For this review, take the finished solid that the model builds, in its own axes (mm). Give positions to 0.01 mm unless a question says otherwise; leave off trailing zeros. Loops run counter-clockwise (first coordinate to the right, second up) from the corner with the lowest first, then second, coordinate; pieces in that order, holes last. Notation, with made-up numbers: (49, 48) -> (55, 48) arc R20 cw to (55, 77) -> close; hole circle Ø11 at (78.5, 19). An arc over 180 degrees is marked (long way). Write each question's results on one line, items separated by ' | '. Start each with the question number.
```python
from build123d import *

# Parameters (mm, degrees)
F1_DEPTH = 60
F2_DEPTH = 50
F3_R     = 39
F4_DEPTH = 10
F3_R_2   = 49
F5_DEPTH = 3
F6_D     = 4
F6_DEPTH = 20
F6_TIP   = 1.2017212381


with BuildPart() as f1:
    # F0 (on Top) → F1 (new body, symmetric)
    with BuildSketch(Plane.XY):
        with BuildLine():
            ThreePointArc((-20.6806279512, -212.5965936405), (-39.6511040787, -210.0990830779), (-51.299249736, -194.9189241108))
            Line((-51.299249736, -194.9189241108), (-96.5925826289, -25.8819045103))
            ThreePointArc((-96.5925826289, -25.8819045103), (-96.7999862455, -25.034315887), (-96.9702211634, -24.1784871615))
            Line((-96.9702211634, -24.1784871615), (-59.4134556551, -237.1734885924))
            ThreePointArc((-59.4134556551, -237.1734885924), (-58.8379861015, -234.2804077793), (-56.4591683744, -232.5361864574))
            Line((-56.4591683744, -232.5361864574), (54.3519994715, -202.8444235207))
            ThreePointArc((54.3519994715, -202.8444235207), (60.4240630584, -198.1851652578), (61.4230672834, -190.5969748068))
            Line((61.4230672834, -190.5969748068), (52.3644007048, -156.7895708867))
            ThreePointArc((52.3644007048, -156.7895708867), (50.8658943672, -168.1718565632), (41.757798987, -175.1607439575))
            Line((41.757798987, -175.1607439575), (-25.8570088532, -193.2780771147))
            ThreePointArc((-25.8570088532, -193.2780771147), (-31.9807332102, -189.7425432088), (-28.4451993043, -183.6188188518))
            Line((-28.4451993043, -183.6188188518), (39.169608536, -165.5014856947))
            ThreePointArc((39.169608536, -165.5014856947), (49.7762102538, -147.1303126238), (31.4050371829, -136.523710906))
            Line((31.4050371829, -136.523710906), (-36.2097706573, -154.6410440632))
            ThreePointArc((-36.2097706573, -154.6410440632), (-42.3334950143, -151.1055101572), (-38.7979611084, -144.9817858003))
            Line((-38.7979611084, -144.9817858003), (28.8168467319, -126.8644526431))
            ThreePointArc((28.8168467319, -126.8644526431), (37.9249421121, -119.8755652488), (39.4234484497, -108.4932795722))
            Line((39.4234484497, -108.4932795722), (9.6592582629, 2.588190451))
            ThreePointArc((9.6592582629, 2.588190451), (5, 8.6602540378), (-2.588190451, 9.6592582629))
            Line((-2.588190451, 9.6592582629), (-79.8622565541, -11.0462653453))
            ThreePointArc((-79.8622565541, -11.0462653453), (-85.934320141, -15.7055236082), (-86.933324366, -23.2937140592))
            Line((-86.933324366, -23.2937140592), (-61.0514198558, -119.8862966881))
            ThreePointArc((-61.0514198558, -119.8862966881), (-56.3921615929, -125.958360275), (-48.8039711418, -126.9573645))
            Line((-48.8039711418, -126.9573645), (23.6404658298, -107.5459361173))
            ThreePointArc((23.6404658298, -107.5459361173), (29.7641901868, -111.0814700232), (26.2286562809, -117.2051943802))
            Line((26.2286562809, -117.2051943802), (-41.3861515594, -135.3225275374))
            ThreePointArc((-41.3861515594, -135.3225275374), (-51.9927532772, -153.6937006083), (-33.6215802063, -164.300302326))
            Line((-33.6215802063, -164.300302326), (33.9932276339, -146.1829691689))
            ThreePointArc((33.9932276339, -146.1829691689), (40.1169519909, -149.7185030748), (36.581418085, -155.8422274318))
            Line((36.581418085, -155.8422274318), (-31.0333897553, -173.9595605889))
            ThreePointArc((-31.0333897553, -173.9595605889), (-41.6399914731, -192.3307336598), (-23.2688184022, -202.9373353776))
            Line((-23.2688184022, -202.9373353776), (44.345989438, -184.8200022204))
            ThreePointArc((44.345989438, -184.8200022204), (50.469713795, -188.3555361264), (46.9341798891, -194.4792604833))
            Line((46.9341798891, -194.4792604833), (-20.6806279512, -212.5965936405))
        make_face()
        with BuildLine():
            Line((-96.5925826289, -25.8819045103), (-51.299249736, -194.9189241108))
            ThreePointArc((-51.299249736, -194.9189241108), (-39.6511040787, -210.0990830779), (-20.6806279512, -212.5965936405))
            Line((-20.6806279512, -212.5965936405), (46.9341798891, -194.4792604833))
            ThreePointArc((46.9341798891, -194.4792604833), (50.469713795, -188.3555361264), (44.345989438, -184.8200022204))
            Line((44.345989438, -184.8200022204), (-23.2688184022, -202.9373353776))
            ThreePointArc((-23.2688184022, -202.9373353776), (-41.6399914731, -192.3307336598), (-31.0333897553, -173.9595605889))
            Line((-31.0333897553, -173.9595605889), (36.581418085, -155.8422274318))
            ThreePointArc((36.581418085, -155.8422274318), (40.1169519909, -149.7185030748), (33.9932276339, -146.1829691689))
            Line((33.9932276339, -146.1829691689), (-33.6215802063, -164.300302326))
            ThreePointArc((-33.6215802063, -164.300302326), (-51.9927532772, -153.6937006083), (-41.3861515594, -135.3225275374))
            Line((-41.3861515594, -135.3225275374), (26.2286562809, -117.2051943802))
            ThreePointArc((26.2286562809, -117.2051943802), (29.7641901868, -111.0814700232), (23.6404658298, -107.5459361173))
            Line((23.6404658298, -107.5459361173), (-48.8039711418, -126.9573645))
            ThreePointArc((-48.8039711418, -126.9573645), (-56.3921615929, -125.958360275), (-61.0514198558, -119.8862966881))
            Line((-61.0514198558, -119.8862966881), (-86.933324366, -23.2937140592))
            ThreePointArc((-86.933324366, -23.2937140592), (-85.934320141, -15.7055236082), (-79.8622565541, -11.0462653453))
            Line((-79.8622565541, -11.0462653453), (-2.588190451, 9.6592582629))
            ThreePointArc((-2.588190451, 9.6592582629), (5, 8.6602540378), (9.6592582629, 2.588190451))
            Line((9.6592582629, 2.588190451), (39.4234484497, -108.4932795722))
            ThreePointArc((39.4234484497, -108.4932795722), (37.9249421121, -119.8755652488), (28.8168467319, -126.8644526431))
            Line((28.8168467319, -126.8644526431), (-38.7979611084, -144.9817858003))
            ThreePointArc((-38.7979611084, -144.9817858003), (-42.3334950143, -151.1055101572), (-36.2097706573, -154.6410440632))
            Line((-36.2097706573, -154.6410440632), (31.4050371829, -136.523710906))
            ThreePointArc((31.4050371829, -136.523710906), (49.7762102538, -147.1303126238), (39.169608536, -165.5014856947))
            Line((39.169608536, -165.5014856947), (-28.4451993043, -183.6188188518))
            ThreePointArc((-28.4451993043, -183.6188188518), (-31.9807332102, -189.7425432088), (-25.8570088532, -193.2780771147))
            Line((-25.8570088532, -193.2780771147), (41.757798987, -175.1607439575))
            ThreePointArc((41.757798987, -175.1607439575), (50.8658943672, -168.1718565632), (52.3644007048, -156.7895708867))
            Line((52.3644007048, -156.7895708867), (61.4230672834, -190.5969748068))
            ThreePointArc((61.4230672834, -190.5969748068), (60.4240630584, -198.1851652578), (54.3519994715, -202.8444235207))
            Line((54.3519994715, -202.8444235207), (-56.4591683744, -232.5361864574))
            ThreePointArc((-56.4591683744, -232.5361864574), (-58.8379861015, -234.2804077793), (-59.4134556551, -237.1734885924))
            ThreePointArc((-59.4134556551, -237.1734885924), (-58.0216629892, -239.5841442033), (-55.4059483937, -240.5361864574))
            Line((-55.4059483937, -240.5361864574), (30.7766323053, -240.5361864574))
            ThreePointArc((30.7766323053, -240.5361864574), (63.8813029697, -224.210769539), (71.0823255463, -188.0087843558))
            Line((71.0823255463, -188.0087843558), (19.3185165258, 5.1763809021))
            ThreePointArc((19.3185165258, 5.1763809021), (10, 17.3205080757), (-5.1763809021, 19.3185165258))
            Line((-5.1763809021, 19.3185165258), (-82.4504470052, -1.3870070824))
            ThreePointArc((-82.4504470052, -1.3870070824), (-94.1418950194, -9.9595314413), (-96.9702211634, -24.1784871615))
            ThreePointArc((-96.9702211634, -24.1784871615), (-96.7999862455, -25.034315887), (-96.5925826289, -25.8819045103))
        make_face()
    extrude(amount=F1_DEPTH, both=True)

    # F0 (on Top) → F2 (cut, symmetric)
    with BuildSketch(Plane.XY):
        with BuildLine():
            ThreePointArc((-20.6806279512, -212.5965936405), (-39.6511040787, -210.0990830779), (-51.299249736, -194.9189241108))
            Line((-51.299249736, -194.9189241108), (-96.5925826289, -25.8819045103))
            ThreePointArc((-96.5925826289, -25.8819045103), (-96.7999862455, -25.034315887), (-96.9702211634, -24.1784871615))
            Line((-96.9702211634, -24.1784871615), (-59.4134556551, -237.1734885924))
            ThreePointArc((-59.4134556551, -237.1734885924), (-58.8379861015, -234.2804077793), (-56.4591683744, -232.5361864574))
            Line((-56.4591683744, -232.5361864574), (54.3519994715, -202.8444235207))
            ThreePointArc((54.3519994715, -202.8444235207), (60.4240630584, -198.1851652578), (61.4230672834, -190.5969748068))
            Line((61.4230672834, -190.5969748068), (52.3644007048, -156.7895708867))
            ThreePointArc((52.3644007048, -156.7895708867), (50.8658943672, -168.1718565632), (41.757798987, -175.1607439575))
            Line((41.757798987, -175.1607439575), (-25.8570088532, -193.2780771147))
            ThreePointArc((-25.8570088532, -193.2780771147), (-31.9807332102, -189.7425432088), (-28.4451993043, -183.6188188518))
            Line((-28.4451993043, -183.6188188518), (39.169608536, -165.5014856947))
            ThreePointArc((39.169608536, -165.5014856947), (49.7762102538, -147.1303126238), (31.4050371829, -136.523710906))
            Line((31.4050371829, -136.523710906), (-36.2097706573, -154.6410440632))
            ThreePointArc((-36.2097706573, -154.6410440632), (-42.3334950143, -151.1055101572), (-38.7979611084, -144.9817858003))
            Line((-38.7979611084, -144.9817858003), (28.8168467319, -126.8644526431))
            ThreePointArc((28.8168467319, -126.8644526431), (37.9249421121, -119.8755652488), (39.4234484497, -108.4932795722))
            Line((39.4234484497, -108.4932795722), (9.6592582629, 2.588190451))
            ThreePointArc((9.6592582629, 2.588190451), (5, 8.6602540378), (-2.588190451, 9.6592582629))
            Line((-2.588190451, 9.6592582629), (-79.8622565541, -11.0462653453))
            ThreePointArc((-79.8622565541, -11.0462653453), (-85.934320141, -15.7055236082), (-86.933324366, -23.2937140592))
            Line((-86.933324366, -23.2937140592), (-61.0514198558, -119.8862966881))
            ThreePointArc((-61.0514198558, -119.8862966881), (-56.3921615929, -125.958360275), (-48.8039711418, -126.9573645))
            Line((-48.8039711418, -126.9573645), (23.6404658298, -107.5459361173))
            ThreePointArc((23.6404658298, -107.5459361173), (29.7641901868, -111.0814700232), (26.2286562809, -117.2051943802))
            Line((26.2286562809, -117.2051943802), (-41.3861515594, -135.3225275374))
            ThreePointArc((-41.3861515594, -135.3225275374), (-51.9927532772, -153.6937006083), (-33.6215802063, -164.300302326))
            Line((-33.6215802063, -164.300302326), (33.9932276339, -146.1829691689))
            ThreePointArc((33.9932276339, -146.1829691689), (40.1169519909, -149.7185030748), (36.581418085, -155.8422274318))
            Line((36.581418085, -155.8422274318), (-31.0333897553, -173.9595605889))
            ThreePointArc((-31.0333897553, -173.9595605889), (-41.6399914731, -192.3307336598), (-23.2688184022, -202.9373353776))
            Line((-23.2688184022, -202.9373353776), (44.345989438, -184.8200022204))
            ThreePointArc((44.345989438, -184.8200022204), (50.469713795, -188.3555361264), (46.9341798891, -194.4792604833))
            Line((46.9341798891, -194.4792604833), (-20.6806279512, -212.5965936405))
        make_face()
    extrude(amount=F2_DEPTH, both=True, mode=Mode.SUBTRACT)

    # F3 (on face) → F4 (cut)
    with BuildSketch(Plane(origin=(19.3185165258, 5.1763809021, 0), x_dir=(-0.2588190451, 0.9659258263, 0), z_dir=(0.9659258263, 0.2588190451, 0))):
        with Locations((-55, 0)):
            Circle(F3_R)
    extrude(amount=-F4_DEPTH, mode=Mode.SUBTRACT)

    # F3 (on face) → F5 (cut)
    with BuildSketch(Plane(origin=(19.3185165258, 5.1763809021, 0), x_dir=(-0.2588190451, 0.9659258263, 0), z_dir=(0.9659258263, 0.2588190451, 0))):
        with Locations((-55, 0)):
            Circle(F3_R_2)
        with Locations((-55, 0)):
            Circle(F3_R, mode=Mode.SUBTRACT)
    extrude(amount=-F5_DEPTH, mode=Mode.SUBTRACT)

    # F6
    with Locations(Plane(origin=(19.3185165258, 5.1763809021, 0), x_dir=(-0.2588190451, 0.9659258263, 0), z_dir=(0.9659258263, 0.2588190451, 0))):
        with Locations((-10, 0), (-32.5, -38.9711431703), (-77.5, -38.9711431703), (-100, 0), (-77.5, 38.9711431703), (-32.5, 38.9711431703)):
            Hole(F6_D / 2, depth=F6_DEPTH)
            with Locations((0, 0, -(F6_DEPTH + F6_TIP / 2))):  # 118° drill point
                Cone(0, F6_D / 2, F6_TIP, mode=Mode.SUBTRACT)


solid = f1.part
```
1. We need section C-C (y = -150). Write out the cut boundary in (x, z), plus the area to 3 significant figures.
2. We need section A-A (x = -16). Write out the cut boundary in (y, z).
3. Draft analysis for pull direction X (two halves, no side actions). For faces 1 (the cylindrical face through (28.64, -54.52, 38.67)), 2 (the flat face through (-14, -108, -60)), 3 (the flat face through (51.314, -114.234, 0.84)), state which applies: released by +X, released by -X, zero draft, split by the parting line, or undercut.
4. Wall thickness on L1, parallel to Z at x = -46.5, y = -157.5; L2, parallel to Y at x = 33, z = 5; L3, parallel to Y at x = 43.5, z = 2: over which ranges is each line inside the solid? List them lowest first.
5. For pin 1 Ø1 at (x, z) = (-71.5, 27.5) entering from +Y; pin 2 Ø2 at (y, z) = (-94, -27) entering from +X; pin 3 Ø10 at (x, z) = (-52.5, -8.5) entering from +Y, all flat-tipped, find the tip position at first contact; note any pin that passes through.
6. We need section B-B (y = -113). Write out the cut boundary in (x, z).
Response:
1) outline: (-74.78, -60) -> (60.9, -60) -> (60.9, 60) -> (-74.78, 60) -> (-74.78, 50) -> (-63.34, 50) -> (-63.34, -50) -> (-74.78, -50) -> close; hole (-52.5, -50) -> (-42.5, -50) -> (-42.5, 50) -> (-52.5, 50) -> close; hole (-18.89, -50) -> (19.75, -50) -> (19.75, 50) -> (-18.89, 50) -> close; hole (40.18, -50) -> (50.25, -50) -> (50.25, 50) -> (40.18, 50) -> close | area: 9,270 mm2
2) outline: (-240.54, -60) -> (16.42, -60) -> (16.42, 60) -> (-240.54, 60) -> close; hole (-221.7, -50) -> (-211.34, -50) -> (-211.34, 50) -> (-221.7, 50) -> close; hole (-200.99, -50) -> (-190.64, -50) -> (-190.64, 50) -> (-200.99, 50) -> close; hole (-180.28, -50) -> (-169.93, -50) -> (-169.93, 50) -> (-180.28, 50) -> close; hole (-159.58, -50) -> (-149.23, -50) -> (-149.23, 50) -> (-159.58, 50) -> close; hole (-138.87, -50) -> (-128.52, -50) -> (-128.52, 50) -> (-138.87, 50) -> close; hole (-118.17, -50) -> (6.07, -50) -> (6.07, 50) -> (-118.17, 50) -> close
3) face 1: undercut | face 2: zero draft | face 3: released by +X
4) L1: z = -60 to -50, 50 to 60 | L2: y = -240.48 to -208.57, -198.21 to -187.86, -177.51 to -167.15, -156.8 to -146.45, -136.19 to -125.02 | L3: y = -238.55 to -205.75, -195.4 to -185.05, -174.58 to -163.56, -138.46 to -95.97
5) pin 1: stops at y = 1.68 | pin 2: stops at x = 46.16 | pin 3: stops at y = 7.98
6) outline: (-81.31, -60) -> (50.98, -60) -> (50.98, 60) -> (-81.31, 60) -> (-81.31, 50) -> (-73.25, 50) -> (-73.25, -50) -> (-81.31, -50) -> close; hole (-62.9, -50) -> (3.29, -50) -> (3.29, 50) -> (-62.9, 50) -> close; hole (29.9, -50) -> (39.92, -50) -> (39.92, 50) -> (29.9, 50) -> close
